Verification items for the finished model (mm, model axes). Face numbers are marked on the shaded views. A direction names the side the tool comes from. Round coordinates to 2 decimals unless told otherwise and drop trailing zeros. Write each loop counter-clockwise with the first axis right and the second up, starting at its lowest first coordinate (ties: lowest second). Pieces come first, ordered by that corner, then holes. Notation, with made-up numbers: M -4.5,45 L 19.5,45 A20 cw 19.5,58 Z; hole C 49,23.5 d9. An arc over 180 degrees is marked long. One line per question, with ' | ' between items.
from build123d import *

# Parameters (mm, degrees)
F1_DEPTH      = 25
F2_R          = 5
F3_R          = 5
F4_R          = 3.2402082651
F5_DEPTH      = 25
F5_DEPTH_BACK = 25
F6_R          = 3.2653549995
F7_DEPTH      = 25
F7_DEPTH_BACK = 25


with BuildPart() as f1:
    # F0 (on Top) → F1 (new body)
    with BuildSketch(Plane.XY):
        Polygon((-23.0555834253, -9.0956758987), (-16.664795906, -4.2834170857), (55.335204094, -4.2834170857), (63.335204094, -4.2834170857), (63.335204094, 4.2834170857), (55.335204094, 4.2834170857), (-16.664795906, 4.2834170857), (-23.0555834253, 9.0956758987), (-32.5767005301, 9.0956758987), (-37.6473867758, 15.2834170857), (-72.6473867758, 15.2834170857), (-76.1434496577, 9.5535986996), (-93.7138741884, 9.5535986996), (-93.7138741884, 7), (-75.9291218825, 7), (-72.9862269919, 11), (-37.9862269919, 11), (-32.9155407462, 4.812258813), (-23.3944236414, 4.812258813), (-17.0036361221, 0), (-23.3944236414, -4.812258813), (-32.9155407462, -4.812258813), (-37.9862269919, -11), (-72.9862269919, -11), (-75.9291218825, -7), (-93.7138741884, -7), (-93.7138741884, -9.5535986996), (-76.1434496577, -9.5535986996), (-72.6473867758, -15.2834170857), (-37.6473867758, -15.2834170857), (-32.5767005301, -9.0956758987), align=None)
    extrude(amount=F1_DEPTH)

    # F2
    f2_edges = [f1.edges().sort_by_distance(p)[0] for p in [
        (63.335204, 0, 25),
        (63.335204, 0, 0),
    ]]
    fillet(f2_edges, radius=F2_R)

    # F3
    f3_edges = [f1.edges().sort_by_distance(p)[0] for p in [
        (-93.713874, 8.276799, 25),
        (-93.713874, 8.276799, 0),
        (-93.713874, -8.276799, 25),
        (-93.713874, -8.276799, 0),
    ]]
    fillet(f3_edges, radius=F3_R)

    # F4 (on face) → F5 (cut, two sides)
    with BuildSketch(Plane.XZ.offset(9.5535986996)) as f5_sk:
        with Locations((-86.387142539, 13.4355006739)):
            Circle(F4_R)
    extrude(amount=F5_DEPTH, mode=Mode.SUBTRACT)
    extrude(f5_sk.sketch, amount=-F5_DEPTH_BACK, mode=Mode.SUBTRACT)

    # F6 (on Front) → F7 (cut, two sides)
    with BuildSketch(Plane.XZ) as f7_sk:
        with Locations((-27.815233916, 13.1105445325)):
            Circle(F6_R)
    extrude(amount=-F7_DEPTH, mode=Mode.SUBTRACT)
    extrude(f7_sk.sketch, amount=F7_DEPTH_BACK, mode=Mode.SUBTRACT)


solid = f1.part
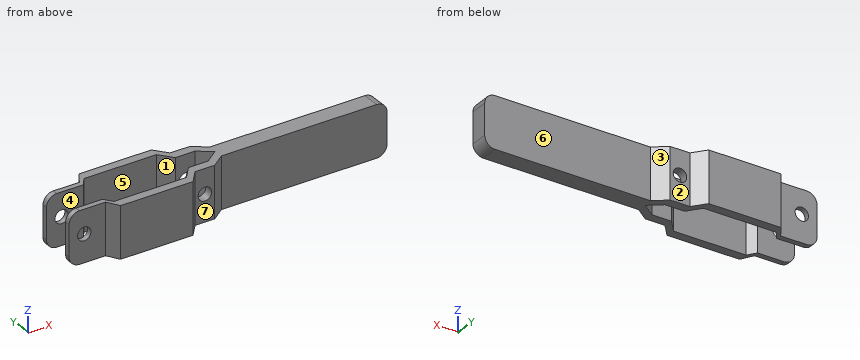
1. Section check C-C, the plane x = 44.5. Record the cut outline in (y, z).
Results:
outline: M -4.28,0 L 4.28,0 L 4.28,25 L -4.28,25 Z
2. Thickness scan on line 1 (Y direction, x = 17, z = 18.5); line 2 (Y direction, x = -21, z = 9); line 3 (Y direction, x = -53, z = 11.25). Record the ranges inside material, lowest first.
Results:
line 1: y = -4.28 to 4.28 | line 2: y = -7.55 to -3.01, 3.01 to 7.55 | line 3: y = -15.28 to -11, 11 to 15.28
3. Tool access check on the marked faces 4, 5, 6 and 7. Record the directions out of +Z, -Z, +X, -X, +Y, -Y that give a thin tool (end or side, any length) a straight path to the whole face; none if there is none.
Results:
face 4: +Z, -Z, -X | face 5: +Z, -Z | face 6: +Z, -Z, +X, +Y | face 7: +Z, -Z, +X, -Y
4. Go/stop test with flat-tipped pins: P1, Ø10.5, axis at x = -29, z = 6.5, coming from the -Y side; P2, Ø10.5, axis at x = -27.5, z = 14.5, coming from the +Y side; P3, Ø1.5, axis at x = 43, z = 17.5, coming from the +Y side; P4, Ø12, axis at y = -10.5, z = 4, coming from the -X side. Record where each tip stops, or that it passes through.
Results:
P1: stops at y = -11.14 | P2: stops at y = 9.31 | P3: stops at y = 4.28 | P4: stops at x = -93.71
5. Section check A-A, the plane x = -59.5. Record the cut outline in (y, z).
Results:
outline: M -15.28,0 L -11,0 L -11,25 L -15.28,25 Z; M 11,0 L 15.28,0 L 15.28,25 L 11,25 Z
6. Mould release check, pull along X, two halves, no side actions. Record for the marked faces 1, 2 and 3: pulls with the +X half, pulls with the -X half, needs draft (parallel to the pull), parting line crosses it, or undercut.
Results:
face 1: undercut | face 2: needs draft | face 3: pulls with the +X half
